Can you work these out from the model? Positions are in its coordinate system, mm. Face numbers are marked on the shaded views. Coordinates: 2 decimals unless noted, no trailing zeros. Order: outer loops, then holes, each group sorted by start corner. A loop starts at its lowest first (then second) coordinate and runs counter-clockwise, first axis right, second up. Notation, with made-up numbers: (25, 57) -> (32, 57) arc R15 ccw to (32, 75) -> close; hole circle Ø11 at (35.5, 44.25). An arc over 180 degrees is marked (long way). Answer in a Markdown table with one row per item.
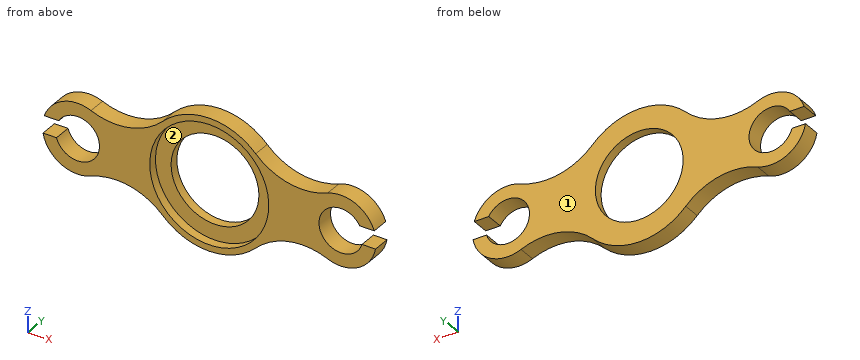
```python
from build123d import *

# Parameters (mm, degrees)
SKETCH6_R           = 50
SKETCH6_R_2         = 25
BOSS_EXTRUDE6_DEPTH = 20
SKETCH6_8_R         = 67.8
CUT_EXTRUDE11_DEPTH = 10
SKETCH9_W           = 21.167456462
SKETCH9_H           = 20
CUT_EXTRUDE13_DEPTH = 30


with BuildPart() as part:
    # Sketch6 → Boss-Extrude6 (new body)
    with BuildSketch(Plane(origin=(0, 0, 0), x_dir=(1, 0, 0), z_dir=(0, 1, 0))):
        with BuildLine():
            ThreePointArc((-52.958333333, -53.107578843), (0, -75), (52.958333333, -53.107578843))
            ThreePointArc((52.958333333, -53.107578843), (91.362529225, -32.640861336), (134.666666667, -36.944402673))
            ThreePointArc((134.666666667, -36.944402673), (190, 0), (134.666666667, 36.944402673))
            ThreePointArc((134.666666667, 36.944402673), (91.362529225, 32.640861336), (52.958333333, 53.107578843))
            ThreePointArc((52.958333333, 53.107578843), (0, 75), (-52.958333333, 53.107578843))
            ThreePointArc((-52.958333333, 53.107578843), (-91.362529225, 32.640861336), (-134.666666667, 36.944402673))
            ThreePointArc((-134.666666667, 36.944402673), (-190, 0), (-134.666666667, -36.944402673))
            ThreePointArc((-134.666666667, -36.944402673), (-91.362529225, -32.640861336), (-52.958333333, -53.107578843))
        make_face()
        with Locations(Location((0, 0, 0), (0, 0, 270))):
            Circle(SKETCH6_R, mode=Mode.SUBTRACT)
        with Locations(Location((150, 0, 0), (0, 0, 270))):
            Circle(SKETCH6_R_2, mode=Mode.SUBTRACT)
        with Locations(Location((-150, 0, 0), (0, 0, 90))):
            Circle(SKETCH6_R_2, mode=Mode.SUBTRACT)
    extrude(amount=BOSS_EXTRUDE6_DEPTH)

    # Sketch6_8 → Cut-Extrude11 (cut)
    with BuildSketch(Plane(origin=(0, 0, 0), x_dir=(1, 0, 0), z_dir=(0, 1, 0))):
        with Locations(Location((0, 0, 0), (0, 0, 270))):
            Circle(SKETCH6_8_R)
    extrude(amount=CUT_EXTRUDE11_DEPTH, mode=Mode.SUBTRACT)

    # Sketch9 → Cut-Extrude13 (cut)
    with BuildSketch(Plane.XZ):
        with Locations((181.273098249, 2.816509548)):
            Rectangle(SKETCH9_W, SKETCH9_H)
        with Locations((-181.273098249, 2.816509548)):
            Rectangle(SKETCH9_W, SKETCH9_H)
    extrude(amount=-CUT_EXTRUDE13_DEPTH, mode=Mode.SUBTRACT)


solid = part.part
```
(1) Suppose I cut it at C-C (x = -150). Please give me the cut outline in (y, z), and give its area (3 significant figures).
Response values:
| item | result |
|---|---|
| outline | (0, -40) -> (20, -40) -> (20, -25) -> (0, -25) -> close; (0, 25) -> (20, 25) -> (20, 40) -> (0, 40) -> close |
| area | 600 mm2 |
(2) Suppose I cut it at D-D (x = 151). Please give me the cut outline in (y, z).
Response values:
| item | result |
|---|---|
| outline | (0, -39.99) -> (20, -39.99) -> (20, -24.98) -> (0, -24.98) -> close; (0, 24.98) -> (20, 24.98) -> (20, 39.99) -> (0, 39.99) -> close |
(3) I need wall thicknesses on line 1 (X direction, y = 16.75, z = 0); line 2 (X direction, y = 7.5, z = 0); line 3 (Z direction, x = -150, y = 13). Which ranges of each line are inside material? Lowest first, please. Write a range as [from, to].
Response values:
| item | result |
|---|---|
| line 1 | [-125, -50], [50, 125] |
| line 2 | [-125, -67.8], [67.8, 125] |
| line 3 | [-40, -25], [25, 40] |
(4) Will these pins go through, and if not, where does the flat tip stop? pin 1 Ø8 at (x, y) = (-183.5, 14.5) entering from -Z; pin 2 Ø7.5 at (x, y) = (-183, 12.5) entering from +Z; pin 3 Ø7.5 at (x, y) = (183.5, 13.5) entering from +Z; pin 4 Ø3 at (x, z) = (88.5, 29) entering from -Y.
Response values:
| item | result |
|---|---|
| pin 1 | z = -27.01 |
| pin 2 | z = 27.28 |
| pin 3 | z = 26.74 |
| pin 4 | y = 0 |
(5) Suppose I cut it at B-B (z = 0). Please give me the cut outline in (x, y), and give its area (3 significant figures).
Response values:
| item | result |
|---|---|
| outline | (-125, 0) -> (-67.8, 0) -> (-67.8, 10) -> (-50, 10) -> (-50, 20) -> (-125, 20) -> close; (50, 10) -> (67.8, 10) -> (67.8, 0) -> (125, 0) -> (125, 20) -> (50, 20) -> close |
| area | 2,640 mm2 |
(6) Suppose I cut it at A-A (x = 0). Please give me the cut outline in (y, z).
Response values:
| item | result |
|---|---|
| outline | (0, -75) -> (20, -75) -> (20, -50) -> (10, -50) -> (10, -67.8) -> (0, -67.8) -> close; (0, 67.8) -> (10, 67.8) -> (10, 50) -> (20, 50) -> (20, 75) -> (0, 75) -> close |
(7) We'd pull the mould along X, two halves only. Please class the marked faces 1 and 2: +X half, -X half, draft (parallel to the pull), parting line (faces both ways), or undercut.
Response values:
| item | result |
|---|---|
| face 1 | draft |
| face 2 | undercut |
